Model file for the job. Use its own axes, mm. A direction names the side the tool comes from. Coordinates: 2 decimals unless noted, no trailing zeros. Order: outer loops, then holes, each group sorted by start corner. A loop starts at its lowest first (then second) coordinate and runs counter-clockwise, first axis right, second up. Notation, with made-up numbers: (40.25, 53) -> (52.25, 53) arc R17 ccw to (52.25, 84) -> close; hole circle Ø1 at (63.5, -37.75). An arc over 180 degrees is marked (long way). Return JSON: item names as keys, results as strings. Group by question number.
1) Which spindle directions (+Z, -Z, +X, -X, +Y, -Y) get a long thin tool onto all of the face, cutting with end or side? Do faces 5 (the flat face through (50, 2, 9)), 6 (the flat face through (34, 5, 10)), 7 (the flat face through (84, 56, 2)). Say none if no direction does.
2) Cut at B-B (z = 2). State how many separate pieces and enclosed holes the cut face has, and give its area (3 significant figures).
3) Probe line 1 (Y direction, x = 74, z = 3); line 2 (X direction, y = 102, z = 1); line 3 (Z direction, x = 40.5, y = 17.5). List the from-to ranges inside material, lowest first.
4) Cut at D-D (x = 22.5). Write the cut outline in (y, z).
5) Cut at C-C (x = 54). Write the cut outline in (y, z).
6) Pull direction Y, two halves, no side cores. Call faces 1 (the cylindrical face through (21.526, 2.465, 11.352)), 2 (the cylindrical face through (53.67, 102.73, 2.46)), 3 (the flat face through (2, 2, 2)), 4 (the cylindrical face through (55.31, 9.54, 2.46)): +Y half, -Y half, draft (parallel to the pull), parting line (faces both ways), or undercut.
7) Flat gauge pins, fed straight in: pin 1 (11.5 mm diameter, centred on x = 15, y = 28.75, fed in from -Z); pin 2 (1.5 mm diameter, centred on y = 1.5, z = 8, fed in from +X); pin 3 (4.5 mm diameter, centred on x = 23, z = 10, fed in from +Y); pin 4 (3 mm diameter, centred on x = 27, y = 84.5, fed in from +Z). Where does each tip first touch, or does it go through?
8) Cut at A-A (y = 28.75). Write the cut outline in (x, z), and give its area (3 significant figures).
from build123d import *

# Parameters (mm, degrees)
SKETCH_R        = 2.5
SKETCH_R_2      = 5
PAD_DEPTH       = 5
CHAMFER_SIZE    = 4
SKETCH001_W     = 32
SKETCH001_H     = 5
PAD001_DEPTH    = 10
SKETCH002_R     = 2
POCKET_DEPTH    = 110.251
CHAMFER001_SIZE = 2


with BuildPart() as part:
    # Sketch → Pad (new body)
    with BuildSketch(Plane.XY):
        Polygon((84, 110.25), (44, 110.25), (0, 53.75), (0, 0), (84, 0), align=None)
        with Locations((15, 45.25)):
            Circle(SKETCH_R, mode=Mode.SUBTRACT)
        with Locations((15, 12.25)):
            Circle(SKETCH_R, mode=Mode.SUBTRACT)
        with Locations((15, 28.75)):
            Circle(SKETCH_R_2, mode=Mode.SUBTRACT)
        with Locations((53, 47)):
            Circle(SKETCH_R, mode=Mode.SUBTRACT)
        with Locations((53, 28.75)):
            Circle(SKETCH_R_2, mode=Mode.SUBTRACT)
        with Locations((53, 10.5)):
            Circle(SKETCH_R, mode=Mode.SUBTRACT)
        with Locations((54, 80.25)):
            Circle(SKETCH_R, mode=Mode.SUBTRACT)
        with Locations((74, 80.25)):
            Circle(SKETCH_R, mode=Mode.SUBTRACT)
        with Locations((54, 100.25)):
            Circle(SKETCH_R, mode=Mode.SUBTRACT)
        with Locations((74, 100.25)):
            Circle(SKETCH_R, mode=Mode.SUBTRACT)
    extrude(amount=PAD_DEPTH)

    # Chamfer
    chamfer_edges = [part.edges().sort_by_distance(p)[0] for p in [
        (0, 0, 2.5),
        (84, 0, 2.5),
    ]]
    chamfer(chamfer_edges, length=CHAMFER_SIZE)

    # Sketch001 (on Face5 of Chamfer) → Pad001 (join)
    with BuildSketch(Plane.XY.offset(5)):
        with Locations((34, 2.5)):
            Rectangle(SKETCH001_W, SKETCH001_H)
    extrude(amount=PAD001_DEPTH)

    # Sketch002 (on Face23 of Pad001) → Pocket (cut, through all)
    with BuildSketch(Plane.XZ):
        with Locations((23, 10)):
            Circle(SKETCH002_R)
        with Locations((45, 10)):
            Circle(SKETCH002_R)
    extrude(amount=-POCKET_DEPTH, mode=Mode.SUBTRACT)

    # Chamfer001
    chamfer001_edges = [part.edges().sort_by_distance(p)[0] for p in [
        (18, 2.5, 15),
        (50, 2.5, 15),
    ]]
    chamfer(chamfer001_edges, length=CHAMFER001_SIZE)


solid = part.part
Answers below:
{
 "1": {"face 5": "+Z, +X, +Y, -Y", "face 6": "+Z, +X, -X, +Y", "face 7": "+Z, -Z, +X, +Y, -Y"},
 "2": {"separate pieces": "1", "enclosed holes": "10", "area": "7,690 mm^2"},
 "3": {"line 1": "y = 0 to 77.75, 82.75 to 97.75, 102.75 to 110.25", "line 2": "x = 37.58 to 52.21, 55.79 to 72.21, 75.79 to 84", "line 3": "z = 0 to 5"},
 "4": {"outline": "(0, 0) -> (82.64, 0) -> (82.64, 5) -> (5, 5) -> (5, 8.06) -> (0, 8.06) -> close; (0, 11.94) -> (5, 11.94) -> (5, 15) -> (0, 15) -> close"},
 "5": {"outline": "(0, 0) -> (8.21, 0) -> (8.21, 5) -> (0, 5) -> close; (12.79, 0) -> (23.85, 0) -> (23.85, 5) -> (12.79, 5) -> close; (33.65, 0) -> (44.71, 0) -> (44.71, 5) -> (33.65, 5) -> close; (49.29, 0) -> (77.75, 0) -> (77.75, 5) -> (49.29, 5) -> close; (82.75, 0) -> (97.75, 0) -> (97.75, 5) -> (82.75, 5) -> close; (102.75, 0) -> (110.25, 0) -> (110.25, 5) -> (102.75, 5) -> close"},
 "6": {"face 1": "draft", "face 2": "undercut", "face 3": "-Y half", "face 4": "undercut"},
 "7": {"pin 1": "stops at z = 0", "pin 2": "stops at x = 50", "pin 3": "stops at y = 5", "pin 4": "stops at z = 5"},
 "8": {"outline": "(0, 0) -> (10, 0) -> (10, 5) -> (0, 5) -> close; (20, 0) -> (48, 0) -> (48, 5) -> (20, 5) -> close; (58, 0) -> (84, 0) -> (84, 5) -> (58, 5) -> close", "area": "320 mm^2"}
}
